Autodesk Inventor part; units mm, degrees
ref_plane "YZ Plane" through (0, 0, 0) normal (1, 0, 0) x (0, 1, 0)
ref_plane "XZ Plane" through (0, 0, 0) normal (0, 1, 0) x (-1, 0, 0)
ref_plane "XY Plane" through (0, 0, 0) normal (0, 0, 1) x (1, 0, 0)
sketch "Boceto1" plane through (0, 0, 0) normal (0, 0, 1) x (1, 0, 0)
  circle A0 centre (0, 0) radius 480
  circle A1 centre (0, 0) radius 125
  dimension "d0" = 960
  dimension "d1" = 250
extrude "Extrusión1" add sketch "Boceto1" against normal blind 25
sketch "Boceto2" plane through (0, 0, 0) normal (0, 0, 1) x (1, 0, 0)
  circle A0 centre (0, 0) radius 325
  circle A1 centre (0, 0) radius 340
  dimension "d4" = 680
  dimension "d5" = 650
extrude "Extrusión2" cut sketch "Boceto2" against normal blind 5
sketch "Boceto3" plane through (0, 0, 0) normal (0, 0, 1) x (1, 0, 0)
  arc A0 (63.1842, 356.4432) -> (-63.1842, 356.4432) centre (0, 0) ccw construction
  arc A1 (65.2787, 368.259) -> (-65.2787, 368.259) centre (0, 0) ccw
  arc A2 (61.0897, 344.6274) -> (-61.0897, 344.6274) centre (0, 0) ccw
  arc A3 (61.0897, 344.6274) -> (65.2787, 368.259) centre (63.1842, 356.4432) ccw
  arc A4 (-65.2787, 368.259) -> (-61.0897, 344.6274) centre (-63.1842, 356.4432) ccw
  line L0 (0, -74.8) -> (0, 448.8)
  point P0 (75, 354.3487)
  point P1 (-75, 354.3487)
  point P2 (0, 362)
  dimension "d8" = 12
  dimension "d9" = 362
  dimension "d15" = 150
extrude "Extrusión3" cut sketch "Boceto3" against normal up to next
sketch "Boceto4" plane through (0, 0, 0) normal (0, 0, 1) x (1, 0, 0)
  circle A0 centre (0, 0) radius 332.5 construction
  circle A1 centre (0, 332.5) radius 6
  dimension "d18" = 665
  dimension "d19" = 12
extrude "Extrusión4" cut sketch "Boceto4" against normal through all
pattern_circular "Patrón circular1" count 18 over 360 about axis through (0, 0, -10) along (0, 0, 1) of "Extrusión4"
properties part number "Brida_1 (flange_1)"
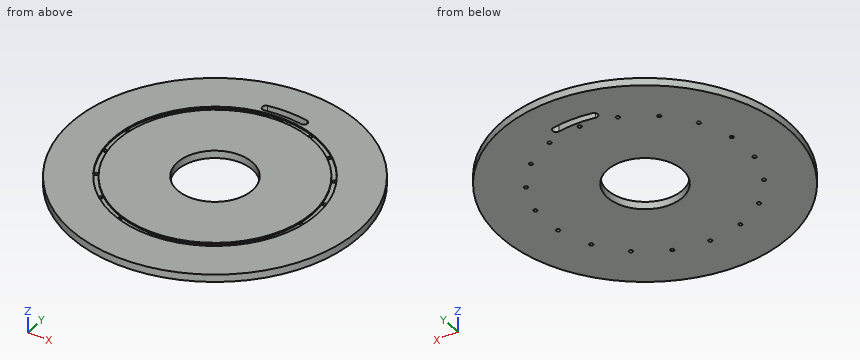
The model under review builds one solid part; all positions refer to its coordinate system, in mm. Round coordinates to 2 decimals unless told otherwise and drop trailing zeros. Order: outer loops, then holes, each group sorted by start corner. A loop starts at its lowest first (then second) coordinate and runs counter-clockwise, first axis right, second up.
(1) For P1, Ø3, axis at x = 39.5, z = -19, coming from the +Y side; P2, Ø11, axis at x = 113.72, y = 312.45, coming from the +Z side; P3, Ø3, axis at y = -58, z = -10, coming from the +X side; P4, Ø3, axis at x = -71, z = -21.5, coming from the +Y side, all flat-tipped, find the tip position at first contact; note any pin that passes through.
Working result:
P1: stops at y = 478.49
P2: passes through
P3: stops at x = 476.66
P4: stops at y = 474.94
(2) Wall thickness on L1, parallel to Y at x = 32.5, z = -14.25; L2, parallel to Y at x = 259, z = -4; L3, parallel to X at y = -55.5, z = -6.5: over which ranges is each line inside the solid? List them lowest first.
Working result:
L1: y = -478.9 to -120.7, 120.7 to 348.49, 372.59 to 478.9
L2: y = -404.13 to -220.27, -196.33 to 196.33, 220.27 to 404.13
L3: x = -476.78 to -333.02, -321.88 to -112, 112 to 321.88, 333.02 to 476.78
(3) Take a section at D-D, the plane y = -185.5. State the section outline as (x, z) points, plus the area to 3 significant figures.
Working result:
outline: (-442.71, -25) - (442.71, -25) - (442.71, 0) - (284.94, 0) - (284.94, -5) - (266.86, -5) - (266.86, 0) - (-266.86, 0) - (-266.86, -5) - (-284.94, -5) - (-284.94, 0) - (-442.71, 0) - close
area: 22,000 mm2
(4) Take a section at B-B, the plane z = -14.75. Count the separate pieces of the cut face and the enclosed holes in it, plus the area to 3 significant figures.
Working result:
separate pieces: 1
enclosed holes: 20
area: 669,000 mm2
(5) Take a section at A-A, the plane y = -79. State the section outline as (x, z) points.
Working result:
outline: (-473.45, -25) - (-96.87, -25) - (-96.87, 0) - (-315.25, 0) - (-315.25, -5) - (-330.69, -5) - (-330.69, 0) - (-473.45, 0) - close; (96.87, -25) - (473.45, -25) - (473.45, 0) - (330.69, 0) - (330.69, -5) - (315.25, -5) - (315.25, 0) - (96.87, 0) - close
(6) Take a section at C-C, the plane x = -159.5. State the section outline as (y, z) points, plus the area to 3 significant figures.
Working result:
outline: (-452.72, -25) - (452.72, -25) - (452.72, 0) - (300.27, 0) - (300.27, -5) - (283.17, -5) - (283.17, 0) - (-283.17, 0) - (-283.17, -5) - (-300.27, -5) - (-300.27, 0) - (-452.72, 0) - close
area: 22,500 mm2
